```python
from build123d import *

# Parameters (mm, degrees)
ESBO_O1_R                = 9
RESSALTO_EXTRUS_O1_DEPTH = 32.5
ESBO_O2_R                = 3
RESSALTO_EXTRUS_O2_DEPTH = 2
FILETE1_R                = 1
ESBO_O4_R                = 5.5
RESSALTO_EXTRUS_O3_DEPTH = 0.4


with BuildPart() as part:
    # Esboço1 → Ressalto-extrusão1 (new body, symmetric)
    with BuildSketch(Plane.XY):
        Circle(ESBO_O1_R)
    extrude(amount=RESSALTO_EXTRUS_O1_DEPTH, both=True)

    # Esboço2 → Ressalto-extrusão2 (add)
    with BuildSketch(Plane.XY.offset(32.5)):
        Circle(ESBO_O2_R)
    extrude(amount=RESSALTO_EXTRUS_O2_DEPTH)

    # Filete1
    filete1_edges = [part.edges().sort_by_distance(p)[0] for p in [
        (-3, 0, 34.5),
    ]]
    fillet(filete1_edges, radius=FILETE1_R)

    # Esboço3 → Corte-Revolução1 (revolve, cut)
    with BuildSketch(Plane(origin=(0, 0, 0), x_dir=(0, 0, -1), z_dir=(1, 0, 0))):
        with BuildLine():
            Line((-29.5, 9), (-25.5, 9))
            ThreePointArc((-25.5, 9), (-27.5, 8.73940243), (-29.5, 9))
        make_face()
    revolve(axis=Axis((0, 0, 34.5), (0, 0, 1)), mode=Mode.SUBTRACT)

    # Esboço4 → Ressalto-extrusão3 (add)
    with BuildSketch(Plane(origin=(0, 0, -32.5), x_dir=(-1, 0, 0), z_dir=(0, 0, -1))):
        Circle(ESBO_O4_R)
    extrude(amount=RESSALTO_EXTRUS_O3_DEPTH)


solid = part.part
```
CAD build for the part. Positions are in the model's coordinates, mm. A direction names the side the tool comes from. Give positions to 0.01 mm unless a question says otherwise; leave off trailing zeros. Write each loop counter-clockwise with the first axis right and the second up, starting at its lowest first coordinate (ties: lowest second). Pieces come first, ordered by that corner, then holes. Notation, with made-up numbers: M 31.5,-5.75 L 42.5,-5.75 A20 cw 42.5,1.25 Z; hole C 32.5,87.5 d1. An arc over 180 degrees is marked long. Return JSON: item names as keys, results as strings. Group by question number.
(1) Drill centre lines: L1, parallel to Z at x = 2.25, y = 6.25; L2, parallel to Z at x = 2, y = -4.5; L3, parallel to X at y = 7, z = 24. Where is each one in solid material? Low to high. Write a range as [from, to].
(2) Band-saw the part on A-A (y = 0). Give the cut face in (x, z).
(3) Band-saw the part on C-C (z = 6.5). Give the cut face in (x, y), and give its area (3 significant figures).
(4) Flat gauge pins, fed straight in: pin 1 Ø3 at (x, y) = (5.5, 6) entering from +Z; pin 2 Ø8 at (x, z) = (7, 8.5) entering from +Y; pin 3 Ø3 at (x, z) = (-2.5, 4) entering from +Y. Where does each tip first touch, or does it go through?
(5) 3-axis set-ups, long thin cutter, end or side, ignore diameter. For faces 1 (the face through (-4, -4, -32.5)), 2 (the face through (0, -4, 32.5)), 3 (the face through (8.584, 2.703, 31.021)): which of +Z, -Z, +X, -X, +Y, -Y reach the whole face in a straight line?
Entries:
{
 "1": {"L1": "z = [-32.5, 32.5]", "L2": "z = [-32.9, 32.5]", "L3": "x = [-5.66, 5.66]"},
 "2": {"outline": "M -9,-32.5 L -5.5,-32.5 L -5.5,-32.9 L 5.5,-32.9 L 5.5,-32.5 L 9,-32.5 L 9,25.5 A7.8 cw 9,29.5 L 9,32.5 L 3,32.5 L 3,33.5 A1 ccw 2,34.5 L -2,34.5 A1 ccw -3,33.5 L -3,32.5 L -9,32.5 L -9,29.5 A7.8 cw -9,25.5 Z"},
 "3": {"outline": "C 0,0 d18", "area": "254 mm^2"},
 "4": {"pin 1": "stops at z = 32.5", "pin 2": "stops at y = 8.49", "pin 3": "stops at y = 8.94"},
 "5": {"face 1": "-Z", "face 2": "+Z", "face 3": "+Z, -Z"}
}
